Part model, mm, in its own coordinate system. A direction names the side the tool comes from. Round coordinates to 2 decimals unless told otherwise and drop trailing zeros. Write each loop counter-clockwise with the first axis right and the second up, starting at its lowest first coordinate (ties: lowest second). Pieces come first, ordered by that corner, then holes.
1) Saw through at C-C on x = -3. Write the cut outline in (y, z), and give its area (3 significant figures).
2) Which spindle directions (+Z, -Z, +X, -X, +Y, -Y) get a long thin tool onto all of the face, cutting with end or side? Do faces 5 (the flat face through (2, 60, 74.5)), 6 (the flat face through (-2, 120, 1)), 7 (the flat face through (-2, 59, -74.5)). Say none if no direction does.
3) Saw through at A-A on y = 107.5. Write the cut outline in (x, z).
4) Flat gauge pin, fed straight in: pin 1 (1 mm diameter, centred on x = -73, z = -40, fed in from -Y). Where does the tip first touch, or does it go through?
5) Drill centre lines: L1, parallel to Y at x = -34.5, z = -3.5; L2, parallel to Z at x = 23, y = 61. Where is each one in solid material? Low to high.
6) Pull direction Y, two halves, no side cores. Call faces 1 (the flat face through (2, 0.5, 1)), 2 (the flat face through (2, 61, 75)), 3 (the flat face through (2, 0, 1)), 4 (the flat face through (-2, 119.5, -1)): +Y half, -Y half, draft (parallel to the pull), parting line (faces both ways), or undercut.
7) Saw through at B-B on z = -63. Write the cut outline in (x, y).
Autodesk Inventor part; units mm, degrees
ref_plane "YZ Plane" through (0, 0, 0) normal (1, 0, 0) x (0, 1, 0)
ref_plane "XZ Plane" through (0, 0, 0) normal (0, 1, 0) x (-1, 0, 0)
ref_plane "XY Plane" through (0, 0, 0) normal (0, 0, 1) x (1, 0, 0)
sketch "Sketch1" plane through (0, 0, 0) normal (0, 1, 0) x (-1, 0, 0)
  line L0 (-120, 75) -> (120, 75)
  line L1 (120, 75) -> (120, -75)
  line L2 (120, -75) -> (-120, -75)
  line L3 (-120, -75) -> (-120, 75)
  line L4 (-120, 75) -> (120, -75) construction
  line L5 (120, 75) -> (-120, -75) construction
  point P0 (0, 0)
  dimension "d0" = 150
  dimension "d1" = 240
extrude "Plate1" add sketch "Sketch1" along normal blind 0.5
sketch "Sketch4" plane through (120, 0, 74.5) normal (0, 0, 1) x (1, 0, 0)
  line L0 (-240, 0) -> (0, 0)
  line L1 (0, 0) -> (0, 120)
  line L2 (0, 120) -> (-240, 120)
  line L3 (-240, 120) -> (-240, 0)
edge flange "Flange1" height 120 angle 90 thickness 0.5 bend radius 0.5 thickness toward (0, 0, 1) relief tear relief width 0.5 relief depth 0.25 edges at (0, 0.5, 75) wall of the first edge with corners at (-120, 0, 74.5) (120, 0, 74.5) (120, 120, 74.5) (-120, 120, 74.5)
bend "Bend1"
corner "Corner1"
sketch "Sketch5" plane through (-120, 0, -74.5) normal (0, 0, -1) x (-1, 0, 0)
  line L0 (-240, 0) -> (0, 0)
  line L1 (0, 0) -> (0, 120)
  line L2 (0, 120) -> (-240, 120)
  line L3 (-240, 120) -> (-240, 0)
edge flange "Flange2" height 120 angle 90 thickness 0.5 bend radius 0.5 thickness toward (0, 0, -1) relief tear relief width 0.5 relief depth 0.25 edges at (0, 0.5, -75) wall of the first edge with corners at (120, 0, -74.5) (-120, 0, -74.5) (-120, 120, -74.5) (120, 120, -74.5)
bend "Bend2"
corner "Corner2"
sketch "Sketch6" plane through (-120, 119.5, -75) normal (0, 1, 0) x (-1, 0, 0)
  line L0 (-240, 0) -> (0, 0)
  line L1 (0, 0) -> (0, 149)
  line L2 (0, 149) -> (-240, 149)
  line L3 (-240, 149) -> (-240, 0)
edge flange "Flange3" height 149 angle 90 thickness 0.5 bend radius 0.5 thickness toward (0, 1, 0) relief tear relief width 0.5 relief depth 0.25 edges at (0, 120, -74.5) wall of the first edge with corners at (120, 119.5, -75) (-120, 119.5, -75) (-120, 119.5, 74) (120, 119.5, 74)
bend "Bend3"
corner "Corner3"
equation "\"d2\" = Thickness"
equation "\"d12\" = BendReliefWidth"
equation "\"d13\" = BendReliefDepth"
equation "\"d14\" = MinimumRemnant"
equation "\"d15\" = TransitionRadius"
equation "\"d18\" = BendRadius"
equation "\"d19\" = CornerReliefSize"
equation "\"d20\" = GapSize"
equation "\"d21\" = JacobiRadiusSize"
equation "\"d22\" = BendReliefWidth"
equation "\"d23\" = BendReliefDepth"
equation "\"d24\" = MinimumRemnant"
equation "\"d25\" = TransitionRadius"
equation "\"d28\" = BendRadius"
equation "\"d29\" = CornerReliefSize"
equation "\"d30\" = GapSize"
equation "\"d31\" = JacobiRadiusSize"
equation "\"d32\" = BendReliefWidth"
equation "\"d33\" = BendReliefDepth"
equation "\"d34\" = MinimumRemnant"
equation "\"d35\" = TransitionRadius"
equation "\"d38\" = BendRadius"
equation "\"d39\" = CornerReliefSize"
equation "\"d40\" = GapSize"
equation "\"d41\" = JacobiRadiusSize"
equation "\"BendRadius\" = Thickness"
equation "\"BendReliefWidth\" = Thickness"
equation "\"BendReliefDepth\" = 0.5 * Thickness"
equation "\"CornerReliefSize\" = 4 * Thickness"
equation "\"MinimumRemnant\" = 2 * Thickness"
equation "\"TransitionRadius\" = BendRadius"
equation "\"JacobiRadiusSize\" = BendRadius"
equation "\"GapSize\" = Thickness"
properties part number "Reflector"
Completed:
1. outline: (0, -74) arc R1 ccw to (1, -75) - (119, -75) arc R1 ccw to (120, -74) - (120, 74) - (119.5, 74) - (119.5, -74) arc R0.5 cw to (119, -74.5) - (1, -74.5) arc R0.5 cw to (0.5, -74) - (0.5, 74) arc R0.5 cw to (1, 74.5) - (120, 74.5) - (120, 75) - (1, 75) arc R1 ccw to (0, 74) - close
1. area: 268 mm2
2. face 5: +X, -X, +Y
2. face 6: +Z, -Z, +X, -X, +Y
2. face 7: +X, -X
3. outline: (-120, -75) - (120, -75) - (120, -74.5) - (-120, -74.5) - close; (-120, 74.5) - (120, 74.5) - (120, 75) - (-120, 75) - close
4. pin 1: stops at y = 0
5. L1: y = 0 to 0.5, 119.5 to 120
5. L2: z = -75 to -74.5, 74.5 to 75
6. face 1: undercut
6. face 2: draft
6. face 3: -Y half
6. face 4: undercut
7. outline: (-120, 0) - (120, 0) - (120, 0.5) - (-120, 0.5) - close; (-120, 119.5) - (120, 119.5) - (120, 120) - (-120, 120) - close
